Drawing for the job (mm, zero at the part's lowest x, y, z). A direction names the side the tool comes from. Coordinates: 2 decimals unless noted, no trailing zeros. Write each loop counter-clockwise with the first axis right and the second up, starting at its lowest first coordinate (ties: lowest second). Pieces come first, ordered by that corner, then holes. Notation, with made-up numbers: (59.25, -37.5) -> (96.25, -37.5) arc R9 ccw to (96.25, -32.5) -> close; hole circle Ø3 at (-3.5, 52.5). An arc over 180 degrees is marked (long way). Answer as CSV lines item,"result".
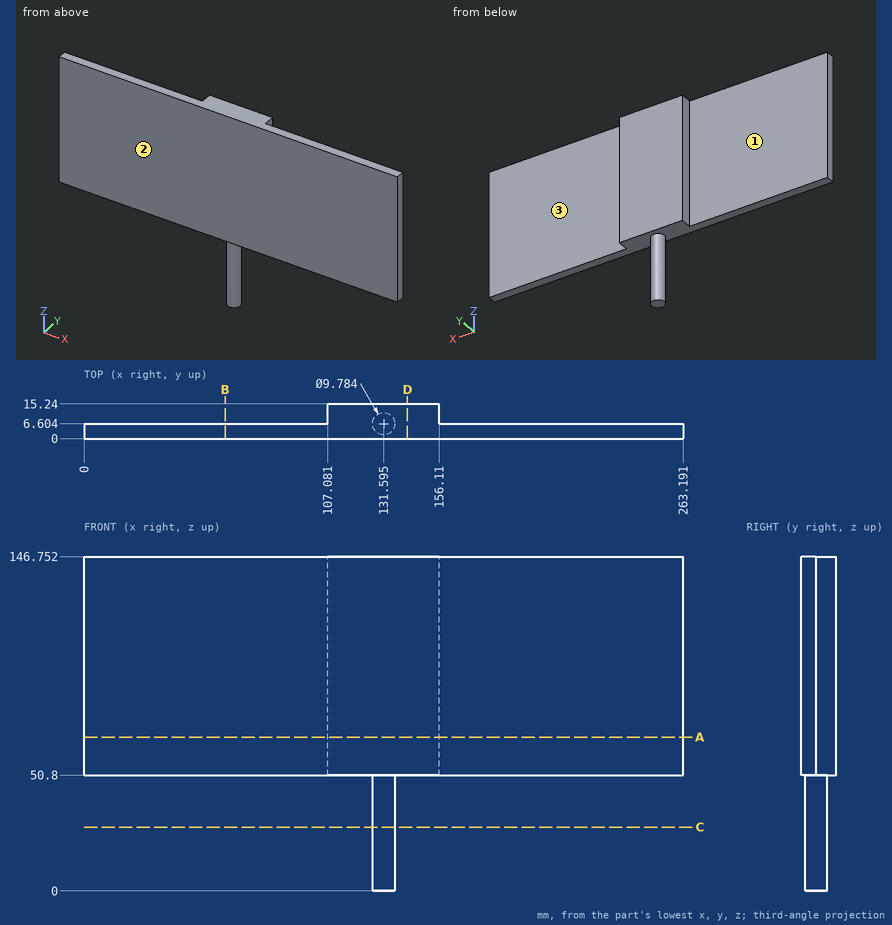
Item 1: Saw through at C-C on z = 28. Give the cut face in (x, y) (1 decimal), and give its area (3 significant figures).
Answer below:
outline,"circle Ø9.8 at (131.6, 6.6)"
area,"75.2 mm2"
Item 2: Wall check: line 1 (Z direction, x = 53, y = 6.5); line 2 (Y direction, x = 166, z = 83); line 3 (X direction, y = 10, z = 128). Give the ranges that are in metal, low to high. Write a range as from..to.
Answer below:
line 1,"z = 50.8..146.75"
line 2,"y = 0..6.6"
line 3,"x = 107.08..156.11"
Item 3: 3-axis set-ups, long thin cutter, end or side, ignore diameter. For the marked faces 1, 2 and 3: which of +Z, -Z, +X, -X, +Y, -Y reach the whole face in a straight line?
Answer below:
face 1,"+Z, -Z, -X, +Y"
face 2,"+Z, -Z, +X, -X, -Y"
face 3,"+Z, -Z, +X, +Y"
Item 4: Saw through at A-A on z = 67.5. Give the cut face in (x, y), and give its area (3 significant figures).
Answer below:
outline,"(0, 0) -> (263.19, 0) -> (263.19, 6.6) -> (156.11, 6.6) -> (156.11, 15.24) -> (107.08, 15.24) -> (107.08, 6.6) -> (0, 6.6) -> close"
area,"2,160 mm2"
Item 5: Saw through at B-B on x = 62. Give the cut face in (y, z).
Answer below:
outline,"(0, 50.8) -> (6.6, 50.8) -> (6.6, 146.75) -> (0, 146.75) -> close"
Item 6: Saw through at D-D on x = 142. Give the cut face in (y, z).
Answer below:
outline,"(0, 50.8) -> (15.24, 50.8) -> (15.24, 146.75) -> (0, 146.75) -> close"
Item 7: Flat gauge pins, fed straight in: pin 1 (4.5 mm diameter, centred on y = 11, z = 86.5, fed in from +X); pin 2 (1.5 mm diameter, centred on x = 69.5, y = 5, fed in from -Z); pin 3 (1 mm diameter, centred on y = 7, z = 28, fed in from -X). Where does each tip first touch, or does it go through?
Answer below:
pin 1,"stops at x = 156.11"
pin 2,"stops at z = 50.8"
pin 3,"stops at x = 126.7"
